Design review of the part built by this model. Coordinates are the model's own, in mm. A direction names the side the tool comes from. Give positions to 0.01 mm unless a question says otherwise; leave off trailing zeros. Order: outer loops, then holes, each group sorted by start corner. A loop starts at its lowest first (then second) coordinate and runs counter-clockwise, first axis right, second up.
```python
from build123d import *

# Parameters (mm, degrees)
EXTRUDE_THIN1_DEPTH = 11
CUT_EXTRUDE1_DEPTH  = 1


with BuildPart() as part:
    # Sketch1 → Extrude-Thin1 (new body)
    with BuildSketch(Plane(origin=(0, 0, 0), x_dir=(1, 0, 0), z_dir=(0, 1, 0))):
        with BuildLine():
            Line((-3, 3), (-3.5, 3))
            ThreePointArc((-3.5, 3), (-3.853553391, 2.853553391), (-4, 2.5))
            Line((-4, 2.5), (-4, 0.5))
            ThreePointArc((-4, 0.5), (-3.853553391, 0.146446609), (-3.5, 0))
            Line((-3.5, 0), (3.5, 0))
            ThreePointArc((3.5, 0), (3.853553391, 0.146446609), (4, 0.5))
            Line((4, 0.5), (4, 2.5))
            ThreePointArc((4, 2.5), (3.853553391, 2.853553391), (3.5, 3))
            Line((3.5, 3), (3, 3))
            Line((3, 3), (3, 2.5))
            Line((3, 2.5), (3.5, 2.5))
            Line((3.5, 2.5), (3.5, 0.5))
            Line((3.5, 0.5), (-3.5, 0.5))
            Line((-3.5, 0.5), (-3.5, 2.5))
            Line((-3.5, 2.5), (-3, 2.5))
            Line((-3, 2.5), (-3, 3))
        make_face()
    extrude(amount=EXTRUDE_THIN1_DEPTH)

    # Sketch3 → Cut-Extrude1 (cut)
    with BuildSketch(Plane.XY):
        with BuildLine():
            Line((-0.5, 6.75), (-0.5, 9.75))
            ThreePointArc((-0.5, 9.75), (0, 10.25), (0.5, 9.75))
            Line((0.5, 9.75), (0.5, 6.75))
            ThreePointArc((0.5, 6.75), (0, 6.25), (-0.5, 6.75))
        make_face()
        with BuildLine():
            Line((0.5, 4.25), (0.5, 1.25))
            ThreePointArc((0.5, 1.25), (0, 0.75), (-0.5, 1.25))
            Line((-0.5, 1.25), (-0.5, 4.25))
            ThreePointArc((-0.5, 4.25), (0, 4.75), (0.5, 4.25))
        make_face()
    extrude(amount=-CUT_EXTRUDE1_DEPTH, mode=Mode.SUBTRACT)


solid = part.part
```
1. Take a section at B-B (x = 0). State the section outline as (y, z) points.
Recorded:
outline: (0, -0.5) - (0.75, -0.5) - (0.75, 0) - (0, 0) - close; (4.75, -0.5) - (6.25, -0.5) - (6.25, 0) - (4.75, 0) - close; (10.25, -0.5) - (11, -0.5) - (11, 0) - (10.25, 0) - close
2. Take a section at C-C (y = 2.25). State the section outline as (x, z) points, then the cut area to 3 significant figures.
Recorded:
outline: (-4, -2.5) arc R0.5 ccw to (-3.5, -3) - (-3, -3) - (-3, -2.5) - (-3.5, -2.5) - (-3.5, -0.5) - (-0.5, -0.5) - (-0.5, 0) - (-3.5, 0) arc R0.5 ccw to (-4, -0.5) - close; (0.5, -0.5) - (3.5, -0.5) - (3.5, -2.5) - (3, -2.5) - (3, -3) - (3.5, -3) arc R0.5 ccw to (4, -2.5) - (4, -0.5) arc R0.5 ccw to (3.5, 0) - (0.5, 0) - close
area: 6.29 mm2
3. For line 1 along X through (y, z) = (9, -1.25); line 2 along X through (y, z) = (10.25, -2.55); line 3 along Z through (x, y) = (3.25, 1.25), list the stretches that pass through material, from the lowest coordinate up.
Recorded:
line 1: x = -4 to -3.5, 3.5 to 4
line 2: x = -4 to -3, 3 to 4
line 3: z = -3 to -2.5, -0.5 to 0
4. Draft analysis for pull direction Z (two halves, no side actions). For faces 1 (the face through (3.5, 5, -2)), 2 (the face through (-0.3, 0, -0.3)), 3 (the face through (0, 5, 0)), state which applies: pulls with the +Z half, pulls with the -Z half, needs draft (parallel to the pull), parting line crosses it, or undercut.
Recorded:
face 1: undercut
face 2: needs draft
face 3: pulls with the +Z half
5. Machinability: for faces 4 (the face through (0, 5, -0.5)), 5 (the face through (-0.3, 11, -0.3)), which of the approach directions +Z, -Z, +X, -X, +Y, -Y give a long, thin tool a straight path to every point of the face, cutting with its end or side? Answer none if there is none.
Recorded:
face 4: +Y, -Y
face 5: +Z, -Z, +X, -X, +Y
6. Take a section at D-D (z = -2.7). State the section outline as (x, y) points, then the cut area to 3 significant figures.
Recorded:
outline: (-3.96, 0) - (-3, 0) - (-3, 11) - (-3.96, 11) - close; (3, 0) - (3.96, 0) - (3.96, 11) - (3, 11) - close
area: 21.1 mm2
7. Take a section at A-A (z = -1.35). State the section outline as (x, y) points, then the cut area to 3 significant figures.
Recorded:
outline: (-4, 0) - (-3.5, 0) - (-3.5, 11) - (-4, 11) - close; (3.5, 0) - (4, 0) - (4, 11) - (3.5, 11) - close
area: 11.0 mm2
8. For pin 1 (0.6 mm diameter, centred on y = 8, z = 0, fed in from -X); pin 2 (0.6 mm diameter, centred on y = 3, z = 0, fed in from +X), all flat-tipped, find the tip position at first contact; note any pin that passes through.
Recorded:
pin 1: stops at x = -3.96
pin 2: stops at x = 3.96
